from build123d import *

# Parameters (mm, degrees)
SKETCH_1_W           = 200
SKETCH_1_H           = 90
EXTRUDE_1_DEPTH      = 8
CUT_EXTRUDE_2_DEPTH  = 206.156038176
SKETCH_7_W           = 200
SKETCH_7_H           = 10
CUT_EXTRUDE_6_DEPTH  = 110.949988631
CUT_EXTRUDE_7_DEPTH  = 110.949988631
EXTRUDE_2_DEPTH      = 20
EXTRUDE_3_DEPTH      = 20
CUT_EXTRUDE_8_DEPTH  = 145.443760826
SKETCH_12_R          = 2
CUT_EXTRUDE_9_DEPTH  = 129.409501341
CUT_EXTRUDE_10_DEPTH = 3


with BuildPart() as part:
    # 草图1 → 凸台-拉伸1 (new body)
    with BuildSketch(Plane.XY):
        Rectangle(SKETCH_1_W, SKETCH_1_H)
    extrude(amount=EXTRUDE_1_DEPTH)

    # 草图3 → 切除-拉伸2 (cut, through all)
    with BuildSketch(Plane.ZY.offset(100)):
        Polygon((0, -45), (8, -15), (8, -45), align=None)
    extrude(amount=-CUT_EXTRUDE_2_DEPTH, mode=Mode.SUBTRACT)

    # 草图7 → 切除-拉伸6 (cut, through all)
    with BuildSketch(Plane(origin=(0, 0, 0), x_dir=(-1, 0, 0), z_dir=(0, 0, -1))):
        with Locations((0, 40)):
            Rectangle(SKETCH_7_W, SKETCH_7_H)
    extrude(amount=-CUT_EXTRUDE_6_DEPTH, mode=Mode.SUBTRACT)

    # 草图8 → 切除-拉伸7 (cut, through all)
    with BuildSketch(Plane(origin=(0, 0, 0), x_dir=(-1, 0, 0), z_dir=(0, 0, -1))):
        with BuildLine():
            Line((60, 35), (-60, 35))
            add(Edge.make_bspline(
                [(60, 35), (0.461478769, -25.014185767), (-60, 35)],
                knots=[0, 0, 0, 1, 1, 1], degree=2))
        make_face()
    extrude(amount=-CUT_EXTRUDE_7_DEPTH, mode=Mode.SUBTRACT)

    # 草图9 → 凸台-拉伸2 (add)
    with BuildSketch(Plane.ZY.offset(100)):
        Polygon((8, -15), (8, 35), (0, 35), (0, -45), align=None)
    extrude(amount=EXTRUDE_2_DEPTH)

    # 草图10 → 凸台-拉伸3 (add)
    with BuildSketch(Plane(origin=(100, 0, 0), x_dir=(0, 0, -1), z_dir=(1, 0, 0))):
        Polygon((0, -45), (0, 35), (-8, 35), (-8, -15), align=None)
    extrude(amount=EXTRUDE_3_DEPTH)

    # 草图11 → 切除-拉伸8 (cut, through all)
    with BuildSketch(Plane(origin=(0, 35, 0), x_dir=(1, 0, 0), z_dir=(0, 1, 0))):
        Polygon((120, 0), (120, -8), (85, -8), align=None)
        Polygon((-120, 0), (-120, -8), (-85, -8), align=None)
    extrude(amount=-CUT_EXTRUDE_8_DEPTH, mode=Mode.SUBTRACT)

    # 草图12 → 切除-拉伸9 (cut, through all)
    with BuildSketch(Plane.XY.offset(8)):
        with Locations((72.7, -9.757802573)):
            Circle(SKETCH_12_R)
        with Locations((-72.7, -9.757802573)):
            Circle(SKETCH_12_R)
        with Locations((72.7, 30)):
            Circle(SKETCH_12_R)
        with Locations((-72.7, 30)):
            Circle(SKETCH_12_R)
    extrude(amount=-CUT_EXTRUDE_9_DEPTH, mode=Mode.SUBTRACT)

    # 草图13 → 切除-拉伸10 (cut)
    with BuildSketch(Plane(origin=(0, 0, 0), x_dir=(-1, 0, 0), z_dir=(0, 0, -1))):
        with BuildLine():
            Line((-59.999999976, 34.999999976), (-100, 35))
            Line((-100, 35), (-100, -25))
            Line((-100, -25), (100, -25))
            Line((100, -25), (100, 35))
            Line((100, 35), (60, 35))
            add(Edge.make_bspline(
                [(60, 35), (0.461478781, -25.014185755), (-59.999999976, 34.999999976)],
                knots=[0, 0, 0, 1, 1, 1], degree=2))
        make_face()
    extrude(amount=-CUT_EXTRUDE_10_DEPTH, mode=Mode.SUBTRACT)


solid = part.part
Geometry check sheet. Reference: the model listing, model coordinates, mm. Give positions to 0.01 mm unless a question says otherwise; leave off trailing zeros. Order: outer loops, then holes, each group sorted by start corner. A loop starts at its lowest first (then second) coordinate and runs counter-clockwise, first axis right, second up.
1) Draft check along X on faces 1 (the flat face through (1, -1, 3)), 2 (the flat face through (83, 35, 4)), 3 (the flat face through (-102.255, 4.449, 4.056)). Enter one of: released by +X, released by -X, zero draft, split by the parting line, or undercut.
Results are:
face 1: undercut
face 2: zero draft
face 3: released by -X
2) Cross-section at C-C (x = -92.5). Record the boundary of the cut face in (y, z).
Results are:
outline: (-45, 0) - (-25, 0) - (-25, 3) - (35, 3) - (35, 6.29) - (-21.43, 6.29) - close
3) Cross-section at B-B (z = 5). Give the number of separate pieces and of enclosed holes in the cut face, then the cut area to 3 significant figures.
Results are:
separate pieces: 1
enclosed holes: 4
area: 9,570 mm2
4) Gauge pin test, flat ends, axial feed: pin 1 (10 mm diameter, centred on x = -62.5, y = -14.5, fed in from -Z); pin 2 (5 mm diameter, centred on x = 72.7, y = 30, fed in from +Z); pin 3 (0.9 mm diameter, centred on x = -42.5, z = 1, fed in from +Y). Record the tip position at first contact, or that the pin passes through.
Results are:
pin 1: stops at z = 3
pin 2: stops at z = 8
pin 3: stops at y = -25
5) Cross-section at A-A (y = 0.5). Record the boundary of the cut face in (x, z), then the cut area to 3 significant figures.
Results are:
outline: (-120, 0) - (-100, 0) - (-100, 3) - (100, 3) - (100, 0) - (120, 0) - (85, 8) - (-85, 8) - close
area: 1,040 mm2
6) Material ranges on probe 1 along Z at (x, y) = (83.5, -10.5); probe 2 along Z at (x, y) = (2, -22), recorded low to high.
Results are:
probe 1: z = 3 to 8
probe 2: z = 3 to 6.13
7) Cross-section at D-D (y = -33). Record the boundary of the cut face in (x, z).
Results are:
outline: (-120, 0) - (120, 0) - (106, 3.2) - (-106, 3.2) - close
